For this review, take the finished solid that the model builds, in its own axes (mm). A direction names the side the tool comes from. Coordinates: 2 decimals unless noted, no trailing zeros. Loops run counter-clockwise (first coordinate to the right, second up) from the corner with the lowest first, then second, coordinate; pieces in that order, holes last. Notation, with made-up numbers: (-8, 60.25) - (9, 60.25) arc R38 cw to (9, 98.25) - close; hole circle Ø10 at (77.5, 60). An arc over 180 degrees is marked (long way). Answer as a JSON object with one key per item and string values. Group by question number.
Item 1: Clearance check with flat-ended pins moving along their axes: pin 1 (1.3 mm diameter, centred on x = 3.5, z = -5, fed in from -Y); pin 2 (2 mm diameter, centred on y = -4, z = -9.5, fed in from -X); pin 3 (1.3 mm diameter, centred on x = -4.5, z = -4.5, fed in from +Y). State where each tip first meets the part, or that it passes through.
Item 2: We need section A-A (z = -7.75). Give the boundary of the cut face in (x, y), then the cut area to 3 significant figures.
Item 3: Tool access review of faces 1 (the flat face through (0, 4, 2.5)), 2 (the flat face through (0, 0, -15)), 3 (the cylindrical face through (5.158, 3.955, 7.24)): name each direction out of +Z, -Z, +X, -X, +Y, -Y from which nothing blocks a thin tool from reaching the whole face with its end or side.
Item 4: We need section C-C (z = -3.5). Give the boundary of the cut face in (x, y), then the cut area to 3 significant figures.
Item 5: We need section B-B (y = 7.5). Give the boundary of the cut face in (x, z).
Item 6: Mouldability with a two-part tool opening along Y and no side actions: class faces 4 (the cylindrical face through (0, 5, 0)), 5 (the conical face through (-0.038, -3.715, -4.178)), 6 (the flat face through (-3.4, 1.7, 3.5)) as released by +Y, released by -Y, zero draft, split by the parting line, or undercut.
Item 7: To check wall thickness, follow line 1 (Z direction, x = -3.75, y = 7); line 2 (Z direction, x = 3.5, y = 2.5); line 3 (X direction, y = -4.75, z = -11.5). State the ranges of each line that lie inside material, in increasing order.
from build123d import *

# Parameters (mm, degrees)
FILLET_2_R               = 3
CUT_EXTRUDE_2_REACH      = 28.287
SKETCH_4_W               = 12.083655217
SKETCH_4_H               = 11.542596028
PATTERN_CIRCULAR_2_COUNT = 4


with BuildPart() as part:
    # ｽｹｯﾁ3 → 回転2 (revolve)
    with BuildSketch(Plane(origin=(0, 0, 0), x_dir=(0, 0, -1), z_dir=(1, 0, 0)), mode=Mode.PRIVATE) as revolve_2_sk:
        Polygon((-1.5, 5), (1.5, 5), (6.5, 6.5), (15, 5.083333333), (15, 0), (13, 0), (13, 3.389079157), (6.629586696, 4.450814707), (1.793537673, 3), (-1.5, 3), (-1.5, 0), (-8, 0), (-8, 6.5), (-6.5, 6.5), (-6.5, 3.5), (-4.5, 3.5), (-4.5, 8), (-3.5, 8), (-3.5, 3.5), (-2.5, 3.5), (-2.5, 9), (-1.5, 9), align=None)
    revolve(revolve_2_sk.sketch.rotate(Axis((0, 0, 0), (0, 0, 1)), 90), axis=Axis((0, 0, 0), (0, 0, 1)))

    # ﾌｨﾚｯﾄ2
    fillet_2_edges = [part.edges().sort_by_distance(p)[0] for p in [
        (5.083333333, 0, -15),
    ]]
    fillet(fillet_2_edges, radius=FILLET_2_R)

    # ｶｯﾄ - 押し出し2: up to this face of the body (flat: up to its plane)
    cut_extrude_2_end = Plane(part.part.faces().sort_by_distance((8.745441559, 0, 1.5))[0])
    # ｽｹｯﾁ4 → ｶｯﾄ - 押し出し2 (cut, up to the picked face)
    with BuildSketch(Plane(origin=(0, 0, -15), x_dir=(-1, 0, 0), z_dir=(0, 0, -1)), mode=Mode.PRIVATE) as cut_extrude_2_sk1:
        with Locations((-8.041827609, 7.771298014)):
            Rectangle(SKETCH_4_W, SKETCH_4_H)
    cut_extrude_2_tool1 = split(extrude(cut_extrude_2_sk1.sketch, amount=-CUT_EXTRUDE_2_REACH, mode=Mode.PRIVATE), bisect_by=cut_extrude_2_end, keep=Keep.BOTH, mode=Mode.PRIVATE)
    cut_extrude_2 = cut_extrude_2_tool1.solids().sort_by(Axis((8.041828, 7.771298, -15), (0, 0, 1)))[0]
    add(cut_extrude_2, mode=Mode.SUBTRACT)

    # 円形ﾊﾟﾀｰﾝ2: ｶｯﾄ - 押し出し2 ×4 about axis
    pattern_circular_2_axis = Axis((0, 0, 0), (0, 0, 1))
    for i in range(1, PATTERN_CIRCULAR_2_COUNT):
        add(cut_extrude_2.rotate(pattern_circular_2_axis, i * 360 / PATTERN_CIRCULAR_2_COUNT), mode=Mode.SUBTRACT)


solid = part.part
Check sheet entries:
{
 "1": {"pin 1": "stops at y = -2", "pin 2": "stops at x = -2", "pin 3": "stops at y = 2"},
 "2": {"outline": "(-5.97, -2) - (-3.77, -2) arc R4.26 cw to (-3.77, 2) - (-5.97, 2) arc R6.29 ccw to start; (-2, -5.97) arc R6.29 ccw to (2, -5.97) - (2, -3.77) arc R4.26 cw to (-2, -3.77) - close; (-2, 3.77) arc R4.26 cw to (2, 3.77) - (2, 5.97) arc R6.29 ccw to (-2, 5.97) - close; (3.77, -2) - (5.97, -2) arc R6.29 ccw to (5.97, 2) - (3.77, 2) arc R4.26 cw to start", "area": "33.3 mm2"},
 "3": {"face 1": "none", "face 2": "-Z, +X, -X, +Y, -Y", "face 3": "+Z"},
 "4": {"outline": "(-5.23, -2) - (-2.89, -2) arc R3.51 cw to (-2.89, 2) - (-5.23, 2) arc R5.6 ccw to start; (-2, -5.23) arc R5.6 ccw to (2, -5.23) - (2, -2.89) arc R3.51 cw to (-2, -2.89) - close; (-2, 2.89) arc R3.51 cw to (2, 2.89) - (2, 5.23) arc R5.6 ccw to (-2, 5.23) - close; (2.89, -2) - (5.23, -2) arc R5.6 ccw to (5.23, 2) - (2.89, 2) arc R3.51 cw to start", "area": "34.7 mm2"},
 "5": {"outline": "(-4.97, 1.5) - (4.97, 1.5) - (4.97, 2.5) - (-4.97, 2.5) - close; (-2.78, 3.5) - (2.78, 3.5) - (2.78, 4.5) - (-2.78, 4.5) - close"},
 "6": {"face 4": "released by +Y", "face 5": "undercut", "face 6": "zero draft"},
 "7": {"line 1": "z = 1.5 to 2.5, 3.5 to 4.5", "line 2": "z = 1.5 to 2.5, 3.5 to 4.5, 6.5 to 8", "line 3": "x = -2 to 2"}
}
